For this review, use the dimensioned drawing (mm, ordinates from the lowest corner) and the shaded views. A direction names the side the tool comes from. Round coordinates to 2 decimals unless told otherwise and drop trailing zeros. Write each loop counter-clockwise with the first axis right and the second up, starting at its lowest first coordinate (ties: lowest second). Pieces come first, ordered by that corner, then holes. Notation, with made-up numbers: (47.5, -35.75) - (78.5, -35.75) arc R25 cw to (78.5, -3.75) - close; hole circle Ø5 at (-6, 60.5). An arc over 180 degrees is marked (long way). Return JSON: item names as keys, results as strings.
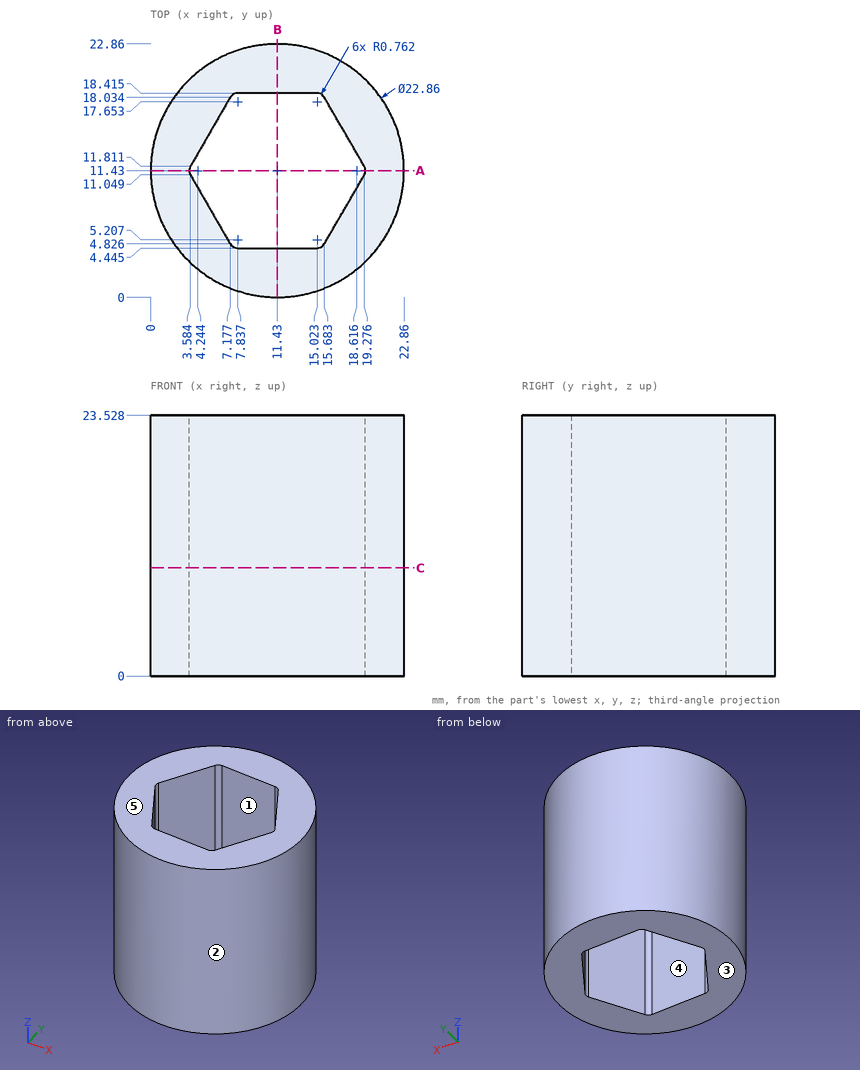
(1) Clearance check with flat-ended pins moving along their axes: pin 1 Ø8 at (y, z) = (5, 8.5) entering from +X; pin 2 Ø2 at (y, z) = (20.5, 5) entering from +X (1 decimal); pin 3 Ø2 at (y, z) = (18.5, 6.5) entering from -X (1 decimal). State where each tip first meets the part, or that it passes through.
Filled in:
{"pin 1": "stops at x = 22.6", "pin 2": "stops at x = 19.5", "pin 3": "stops at x = 1.7"}
(2) Add section C-C (z = 9.75). Write out the cut boundary in (x, y) (1 decimal).
Filled in:
{"outline": "circle Ø22.9 at (11.4, 11.4); hole (3.6, 11) - (7.2, 4.8) arc R0.8 ccw to (7.8, 4.4) - (15, 4.4) arc R0.8 ccw to (15.7, 4.8) - (19.3, 11) arc R0.8 ccw to (19.3, 11.8) - (15.7, 18) arc R0.8 ccw to (15, 18.4) - (7.8, 18.4) arc R0.8 ccw to (7.2, 18) - (3.6, 11.8) arc R0.8 ccw to start"}
(3) Mouldability with a two-part tool opening along Y and no side actions: class the marked faces 1, 2 and 3 as released by +Y, released by -Y, zero draft, split by the parting line, or undercut.
Filled in:
{"face 1": "undercut", "face 2": "split by the parting line", "face 3": "zero draft"}
(4) For the marked faces 4 and 5, list the 3-axis set-ups (+Z, -Z, +X, -X, +Y, -Y) from which the entire face can be reached by the end or side of a thin tool; tool diameter is ignored.
Filled in:
{"face 4": "+Z, -Z", "face 5": "+Z, +X, -X, +Y, -Y"}
(5) Add section B-B (x = 11.43). Write out the cut boundary in (y, z) (1 decimal).
Filled in:
{"outline": "(0, 0) - (4.4, 0) - (4.4, 23.5) - (0, 23.5) - close; (18.4, 0) - (22.9, 0) - (22.9, 23.5) - (18.4, 23.5) - close"}
(6) Wall thickness on line 1 (X direction, y = 11.5, z = 1) (1 decimal); line 2 (X direction, y = 17.25, z = 20.5) (1 decimal); line 3 (Y direction, x = 4.75, z = 15.5) (1 decimal): over which ranges is each line inside the solid? List them lowest first.
Filled in:
{"line 1": "x = 0 to 3.5, 19.4 to 22.9", "line 2": "x = 1.6 to 6.7, 16.1 to 21.3", "line 3": "y = 2.2 to 9, 13.8 to 20.7"}
(7) Add section A-A (y = 11.43). Write out the cut boundary in (x, z), plus the area to 3 significant figures.
Filled in:
{"outline": "(0, 0) - (3.48, 0) - (3.48, 23.53) - (0, 23.53) - close; (19.38, 0) - (22.86, 0) - (22.86, 23.53) - (19.38, 23.53) - close", "area": "164 mm2"}
